from build123d import *

# Parameters (mm, degrees)
F1_DEPTH = 4.1148
F2_R     = 2.9464
F3_DEPTH = 50.8
F4_SIZE2 = 5.08
F4_SIZE  = 2.54


with BuildPart() as f1:
    # F0 (on Top) → F1 (new body)
    with BuildSketch(Plane.XY):
        Polygon((3.1593841377, -5.4911205733), (6.3351419806, -0.0094533631), (3.1757578428, 5.4816672102), (-3.1593841377, 5.4911205733), (-6.3351419806, 0.0094533631), (-3.1757578428, -5.4816672102), align=None)
    extrude(amount=F1_DEPTH)

    # F2 (on face) → F3 (join)
    with BuildSketch(Plane(origin=(0, 0, 0), x_dir=(1, 0, 0), z_dir=(0, 0, -1))):
        Circle(F2_R)
    extrude(amount=F3_DEPTH)

    # F4
    f4_edges = [f1.edges().sort_by_distance(p)[0] for p in [
        (-2.9464, 0, -50.8),
    ]]
    f4_side = f1.faces().sort_by_distance((0, 0, -50.8))[0]
    chamfer(f4_edges, length=F4_SIZE, length2=F4_SIZE2, reference=f4_side)


solid = f1.part
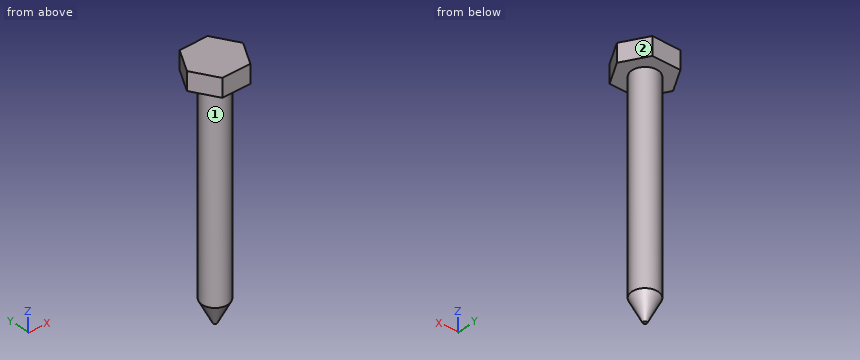
Model file for the job. Use its own axes, mm. Face numbers are marked on the shaded views. A direction names the side the tool comes from. Give positions to 0.01 mm unless a question says otherwise; leave off trailing zeros. Write each loop counter-clockwise with the first axis right and the second up, starting at its lowest first coordinate (ties: lowest second). Pieces come first, ordered by that corner, then holes. Notation, with made-up numbers: (21, -6) - (59, -6) arc R14 cw to (59, 18) - close; hole circle Ø8 at (73.25, 2.5). An arc over 180 degrees is marked (long way). Answer as CSV lines item,"result".
1. Drill centre lines: L1, parallel to Z at x = -2.5, y = -3.5; L2, parallel to Y at x = -0.25, z = 0.5; L3, parallel to Y at x = 0.25, z = -31. Where is each one in solid material? Low to high. Write a range as [from, to].
Responses:
L1,"z = [0, 4.11]"
L2,"y = [-5.49, 5.49]"
L3,"y = [-2.94, 2.94]"
2. Band-saw the part on C-C (x = -4). Write the cut outline in (y, z).
Responses:
outline,"(-4.05, 0) - (4.04, 0) - (4.04, 4.11) - (-4.05, 4.11) - close"
3. 3-axis set-ups, long thin cutter, end or side, ignore diameter. For the marked faces 1 and 2: which of +Z, -Z, +X, -X, +Y, -Y reach the whole face in a straight line?
Responses:
face 1,"-Z"
face 2,"+Z, -Z, +X, +Y"
4. Band-saw the part on A-A (z = -29). Write the cut outline in (x, y), and give its area (3 significant figures).
Responses:
outline,"circle Ø5.89 at (0, 0)"
area,"27.3 mm2"
5. Pin check, flat tips, straight feed: pin 1 (1 mm diameter, centred on x = -2.5, z = -4.5, fed in from -Y); pin 2 (5 mm diameter, centred on x = -3, y = 1.5, fed in from -Z); pin 3 (5 mm diameter, centred on y = -3.5, z = -30.5, fed in from -X). Stop position of each tip, or through.
Responses:
pin 1,"stops at y = -2.16"
pin 2,"stops at z = -49.9"
pin 3,"stops at x = -2.77"
6. Band-saw the part on B-B (y = -4). Write the cut outline in (x, z).
Responses:
outline,"(-4.03, 0) - (4.02, 0) - (4.02, 4.11) - (-4.03, 4.11) - close"
